Autodesk Inventor part; units mm, degrees
ref_plane "YZ Plane" through (0, 0, 0) normal (1, 0, 0) x (0, 1, 0)
ref_plane "XZ Plane" through (0, 0, 0) normal (0, 1, 0) x (-1, 0, 0)
ref_plane "XY Plane" through (0, 0, 0) normal (0, 0, 1) x (1, 0, 0)
sketch "Sketch1" plane through (0, 0, 0) normal (0, 0, 1) x (1, 0, 0)
  line L0 (0, 0) -> (10, 0)
  line L1 (10, 0) -> (10, -10)
  line L2 (10, -10) -> (0, -10)
  line L3 (0, -10) -> (0, 0)
  dimension "d0" = 10
  dimension "d1" = 10
extrude "Extrusion1" add sketch "Sketch1" along normal blind 1.5
sketch "Sketch2" plane through (1.5, -10, 0) normal (-1, 0, 0) x (0, -1, 0)
  line L0 (-10, 0) -> (0, 0)
  line L1 (0, 0) -> (0, 10)
  line L2 (0, 10) -> (-10, 10)
  line L3 (-10, 10) -> (-10, 0)
edge flange "Flange1" height 10 angle 90 thickness 1.5 bend radius 1.5 thickness toward (-1, 0, 0) relief tear relief width 1.5 relief depth 0.75 edges at (0, -5, 1.5) wall of the first edge with corners at (1.5, 0, 0) (1.5, -10, 0) (1.5, -10, 10) (1.5, 0, 10)
bend "Bend1"
corner "Corner1"
sketch "Sketch3" plane through (0, -10, 10) normal (-1, 0, 0) x (0, 0, 1)
  circle A0 centre (-3.5, 5) radius 1
  line L0 (0, 10) -> (0, 0)
  line L1 (-7, 10) -> (0, 10)
  point P0 (-10, 10)
  dimension "d15" = 2
  dimension "d16" = 3.5
  dimension "d17" = 5
extrude "Extrusion2" add sketch "Sketch3" along normal blind 0.1
sketch "Sketch4" plane through (0, 0, 0) normal (0, 0, -1) x (-1, 0, 0)
  circle A0 centre (-6.5, -5) radius 1
  line L0 (-10, -10) -> (-3, -10)
  line L1 (-10, 0) -> (-10, -10)
  point P0 (0, 0)
  dimension "d20" = 2
  dimension "d21" = 5
  dimension "d22" = 3.5
extrude "Extrusion3" add sketch "Sketch4" against normal blind 1.6
sketch "Sketch5" plane through (0, 0, 1.5) normal (0, 0, 1) x (1, 0, 0)
  line L0 (3, 0) -> (3, -10)
  circle A0 centre (6.5, -5) radius 1
  point P0 (0, 0)
equation "\"d4\" = Thickness"
equation "\"d5\" = BendReliefWidth"
equation "\"d6\" = BendReliefDepth"
equation "\"d7\" = MinimumRemnant"
equation "\"d8\" = TransitionRadius"
equation "\"d11\" = BendRadius"
equation "\"d12\" = CornerReliefSize"
equation "\"d13\" = GapSize"
equation "\"d14\" = JacobiRadiusSize"
equation "\"BendRadius\" = Thickness"
equation "\"BendReliefWidth\" = Thickness"
equation "\"BendReliefDepth\" = 0.5 * Thickness"
equation "\"CornerReliefSize\" = 4 * Thickness"
equation "\"MinimumRemnant\" = 2 * Thickness"
equation "\"TransitionRadius\" = BendRadius"
equation "\"JacobiRadiusSize\" = BendRadius"
equation "\"GapSize\" = Thickness"
properties part number "center_joint"
Could you check a few things on this model? Use its own coordinates, in mm. A direction names the side the tool comes from. Coordinates: 2 decimals unless noted, no trailing zeros. Loops run counter-clockwise (first coordinate to the right, second up) from the corner with the lowest first, then second, coordinate; pieces in that order, holes last.
1) Imagine slicing it at A-A (x = 6.5). List the corners of the cut face in (y, z) for me.
Reported:
outline: (-10, 0) - (0, 0) - (0, 1.5) - (-4, 1.5) - (-4, 1.6) - (-6, 1.6) - (-6, 1.5) - (-10, 1.5) - close
2) Please list where these lines run through material, in increasing order: line 1 along X through (y, z) = (-7.5, 4.75); line 2 along Z through (x, y) = (6.75, -5).
Reported:
line 1: x = 0 to 1.5
line 2: z = 0 to 1.6
3) Imagine slicing it at D-D (y = -3.25). List the corners of the cut face in (x, z) for me, and give its area (3 significant figures).
Reported:
outline: (0, 3) arc R3 ccw to (3, 0) - (10, 0) - (10, 1.5) - (3, 1.5) arc R1.5 cw to (1.5, 3) - (1.5, 10) - (0, 10) - close
area: 26.3 mm2
4) Which directions (+Z, -Z, +X, -X, +Y, -Y) give clear straight access to the entire face, cutting with the end or side of a thin tool? Please do faces 1 (the face through (1.5, -5, 6)), 2 (the face through (-0.1, -5, 6)).
Reported:
face 1: +Z, +X, +Y, -Y
face 2: +Z, -Z, -X, +Y, -Y
5) Will these pins go through, and if not, where does the flat tip stop? pin 1 Ø2 at (y, z) = (-4.5, 7) entering from +X; pin 2 Ø1.6 at (x, y) = (6.5, -4.5) entering from +Z.
Reported:
pin 1: stops at x = 1.5
pin 2: stops at z = 1.6
6) Imagine slicing it at B-B (y = -5). List the corners of the cut face in (x, z) for me, and give its area (3 significant figures).
Reported:
outline: (-0.1, 5.5) - (0, 5.5) - (0, 3) arc R3 ccw to (3, 0) - (10, 0) - (10, 1.5) - (7.5, 1.5) - (7.5, 1.6) - (5.5, 1.6) - (5.5, 1.5) - (3, 1.5) arc R1.5 cw to (1.5, 3) - (1.5, 10) - (0, 10) - (0, 7.5) - (-0.1, 7.5) - close
area: 26.7 mm2
7) Imagine slicing it at C-C (z = 7.75). List the corners of the cut face in (x, y) for me.
Reported:
outline: (0, -10) - (1.5, -10) - (1.5, 0) - (0, 0) - close
